The listing builds one solid part. Answer for the finished solid, in the listing's coordinates (mm). Face numbers are marked on the shaded views. Give positions to 0.01 mm unless a question says otherwise; leave off trailing zeros. Write each loop counter-clockwise with the first axis right and the second up, starting at its lowest first coordinate (ties: lowest second). Pieces come first, ordered by that corner, then holes. Notation, with made-up numbers: (-27.5, 71.5) -> (30.5, 71.5) arc R14 ccw to (30.5, 78.5) -> close; hole circle Ø1 at (72, 67). An arc over 180 degrees is marked (long way). Write each question's results on one line, items separated by ' | '. Start each with the question number.
Autodesk Inventor part; units mm, degrees
ref_plane "YZ Plane" through (0, 0, 0) normal (1, 0, 0) x (0, 1, 0)
ref_plane "XZ Plane" through (0, 0, 0) normal (0, 1, 0) x (-1, 0, 0)
ref_plane "XY Plane" through (0, 0, 0) normal (0, 0, 1) x (1, 0, 0)
sketch "スケッチ1" plane through (0, 0, 0) normal (0, 0, 1) x (1, 0, 0)
  line L0 (0, 0) -> (70, 0)
  line L1 (70, 0) -> (70, -42.5)
  line L2 (70, -42.5) -> (0, -42.5)
  line L3 (0, -42.5) -> (0, 0)
  dimension "d0" = 70
  dimension "d1" = 42.5
extrude "押し出し1" add sketch "スケッチ1" along normal blind 5.5
sketch "スケッチ2" plane through (0, 0, 5.5) normal (0, 0, 1) x (1, 0, 0)
  line L0 (4.5, -38) -> (65.5, -38)
  line L1 (65.5, -38) -> (65.5, -4.5)
  line L2 (65.5, -4.5) -> (4.5, -4.5)
  line L3 (4.5, -4.5) -> (4.5, -38)
  line L4 (0, 0) -> (0, -42.5)
  line L5 (0, -42.5) -> (70, -42.5)
  dimension "d4" = 61
  dimension "d5" = 33.5
  dimension "d6" = 4.5
  dimension "d7" = 4.5
hole "穴1" at (4.5, -38, 5.5) at (4.5, -4.5, 5.5) at (65.5, -4.5, 5.5) at (65.5, -38, 5.5) direction (0, 0, -1) diameter 3 end through all
fillet "フィレット1" radius 4.5 4 edges at (0, 0, 2.75) (70, 0, 2.75) (70, -42.5, 2.75) (0, -42.5, 2.75)
sketch "スケッチ3" plane through (0, 0, 5.5) normal (0, 0, 1) x (1, 0, 0)
  line L0 (65.5, 0) -> (4.5, 0)
  line L1 (70, -38) -> (70, -4.5)
  point P0 (0, 0)
  point P1 (46, -23.5)
  dimension "d16" = 23.5
  dimension "d17" = 24
hole "穴2" at (46, -23.5, 5.5) direction (0, 0, -1) diameter 17 end through all
sketch "スケッチ4" plane through (0, 0, 0) normal (0, 0, -1) x (-1, 0, 0)
  line L0 (-4.5, -42.5) -> (-65.5, -42.5)
  line L1 (0, -4.5) -> (0, -38)
  point P0 (0, 0)
  point P1 (-10, -35.5)
  point P2 (-10, -30)
  point P3 (-10, -24.5)
  point P4 (-10, -19)
  point P5 (-10, -13.5)
  point P6 (-10, -8)
  point P7 (-15.5, -35.5)
  point P8 (-15.5, -30)
  point P9 (-15.5, -24.5)
  point P10 (-15.5, -19)
  point P11 (-15.5, -13.5)
  point P12 (-15.5, -8)
  point P13 (-21, -35.5)
  point P14 (-21, -30)
  point P15 (-21, -24.5)
  point P16 (-21, -19)
  point P17 (-21, -13.5)
  point P18 (-21, -8)
  point P19 (-26.5, -35.5)
  point P20 (-26.5, -30)
  point P21 (-26.5, -24.5)
  point P22 (-26.5, -19)
  point P23 (-26.5, -13.5)
  point P24 (-26.5, -8)
  point P25 (-32, -35.5)
  point P26 (-32, -30)
  point P27 (-32, -24.5)
  point P28 (-32, -19)
  point P29 (-32, -13.5)
  point P30 (-32, -8)
  dimension "d25" = 7
  dimension "d26" = 10
  dimension "d29" = 5.5
  dimension "d32" = 5.5
hole "穴3" at (10, -35.5, 0) at (10, -30, 0) at (10, -24.5, 0) at (10, -19, 0) at (10, -13.5, 0) at (10, -8, 0) at (15.5, -35.5, 0) at (15.5, -30, 0) at (15.5, -24.5, 0) at (15.5, -19, 0) at (15.5, -13.5, 0) at (15.5, -8, 0) at (21, -35.5, 0) at (21, -30, 0) at (21, -24.5, 0) at (21, -19, 0) at (21, -13.5, 0) at (21, -8, 0) at (26.5, -35.5, 0) at (26.5, -30, 0) at (26.5, -24.5, 0) at (26.5, -19, 0) at (26.5, -13.5, 0) at (26.5, -8, 0) at (32, -35.5, 0) at (32, -30, 0) at (32, -24.5, 0) at (32, -19, 0) at (32, -13.5, 0) at (32, -8, 0) direction (0, 0, 1) diameter 4.5 end through all
properties part number "ロボット回転t5.5_2" material "木材 (カエデ材)"
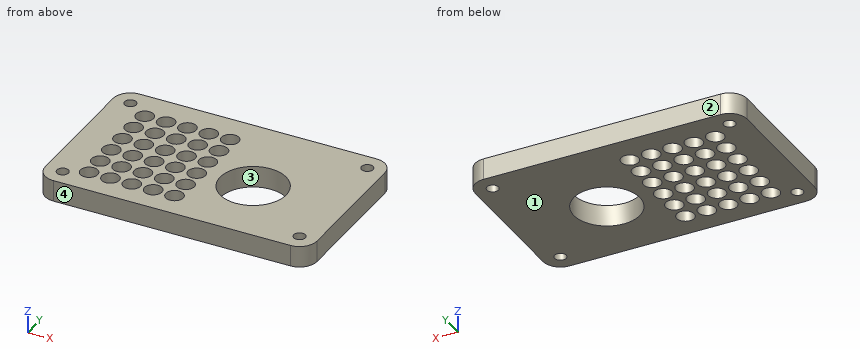
1. The mould has two halves that part along Y. Classify the marked faces 1, 2, 3 and 4: pulls with the +Y half, pulls with the -Y half, needs draft (parallel to the pull), parting line crosses it, or undercut.
2. Section D-D (z = 4.7) is taken. Give the number of separate pieces and of enclosed holes in the cut face, then the cut area to 3 significant figures.
3. Consider probe 1 along X at (y, z) = (-8, 1.65); probe 2 along X at (y, z) = (-38, 0.7); probe 3 along Y at (x, z) = (4.5, 4.75). Determine where each line is inside the solid, lowest interval first. Write a range as [from, to].
4. Section C-C (y = -19) is taken. Write down the section's boundary in (x, z).
5. Section B-B (x = 15.5) is taken. Write down the section's boundary in (y, z).
6. Section A-A (y = -8) is taken. Write down the section's boundary in (x, z), then the cut area to 3 significant figures.
Results:
1) face 1: needs draft | face 2: pulls with the +Y half | face 3: undercut | face 4: pulls with the -Y half
2) separate pieces: 1 | enclosed holes: 35 | area: 2,230 mm²
3) probe 1: x = [0, 7.75], [12.25, 13.25], [17.75, 18.75], [23.25, 24.25], [28.75, 29.75], [34.25, 70] | probe 2: x = [0, 3], [6, 64], [67, 70] | probe 3: y = [-42.5, -39.5], [-36.5, -6], [-3, 0]
4) outline: (0, 0) -> (7.75, 0) -> (7.75, 5.5) -> (0, 5.5) -> close; (12.25, 0) -> (13.25, 0) -> (13.25, 5.5) -> (12.25, 5.5) -> close; (17.75, 0) -> (18.75, 0) -> (18.75, 5.5) -> (17.75, 5.5) -> close; (23.25, 0) -> (24.25, 0) -> (24.25, 5.5) -> (23.25, 5.5) -> close; (28.75, 0) -> (29.75, 0) -> (29.75, 5.5) -> (28.75, 5.5) -> close; (34.25, 0) -> (38.79, 0) -> (38.79, 5.5) -> (34.25, 5.5) -> close; (53.21, 0) -> (70, 0) -> (70, 5.5) -> (53.21, 5.5) -> close
5) outline: (-42.5, 0) -> (-37.75, 0) -> (-37.75, 5.5) -> (-42.5, 5.5) -> close; (-33.25, 0) -> (-32.25, 0) -> (-32.25, 5.5) -> (-33.25, 5.5) -> close; (-27.75, 0) -> (-26.75, 0) -> (-26.75, 5.5) -> (-27.75, 5.5) -> close; (-22.25, 0) -> (-21.25, 0) -> (-21.25, 5.5) -> (-22.25, 5.5) -> close; (-16.75, 0) -> (-15.75, 0) -> (-15.75, 5.5) -> (-16.75, 5.5) -> close; (-11.25, 0) -> (-10.25, 0) -> (-10.25, 5.5) -> (-11.25, 5.5) -> close; (-5.75, 0) -> (0, 0) -> (0, 5.5) -> (-5.75, 5.5) -> close
6) outline: (0, 0) -> (7.75, 0) -> (7.75, 5.5) -> (0, 5.5) -> close; (12.25, 0) -> (13.25, 0) -> (13.25, 5.5) -> (12.25, 5.5) -> close; (17.75, 0) -> (18.75, 0) -> (18.75, 5.5) -> (17.75, 5.5) -> close; (23.25, 0) -> (24.25, 0) -> (24.25, 5.5) -> (23.25, 5.5) -> close; (28.75, 0) -> (29.75, 0) -> (29.75, 5.5) -> (28.75, 5.5) -> close; (34.25, 0) -> (70, 0) -> (70, 5.5) -> (34.25, 5.5) -> close | area: 261 mm²
